For this review, take the finished solid that the model builds, in its own axes (mm). Give positions to 0.01 mm unless a question says otherwise; leave off trailing zeros. Write each loop counter-clockwise with the first axis right and the second up, starting at its lowest first coordinate (ties: lowest second). Pieces come first, ordered by that corner, then holes. Notation, with made-up numbers: (58.25, -22) -> (77.25, -22) arc R4 cw to (77.25, -18) -> close; hole circle Ø9 at (32.25, 35). An arc over 180 degrees is marked (long way). Return JSON: item names as keys, results as strings.
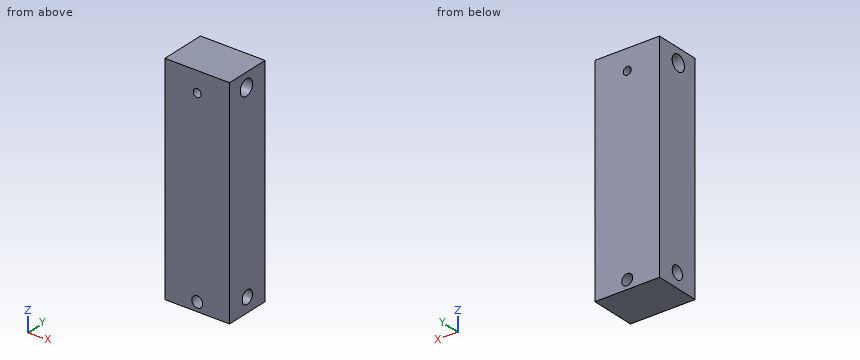
from build123d import *

# Parameters (mm, degrees)
SKETCH_1_W          = 34.660183122
SKETCH_1_H          = 24.57042631
EXTRUDE_1_DEPTH     = 117
SKETCH_2_R          = 2.936506095
SKETCH_2_R_2        = 2.138363717
CUT_EXTRUDE_1_DEPTH = 117
SKETCH_3_R          = 4.242126228
CUT_EXTRUDE_2_DEPTH = 117
SKETCH_4_R          = 3.532728848
CUT_EXTRUDE_3_DEPTH = 50


with BuildPart() as part:
    # 草图1 → 凸台-拉伸1 (new body)
    with BuildSketch(Plane.XY):
        with Locations((17.330091561, 12.285213155)):
            Rectangle(SKETCH_1_W, SKETCH_1_H)
    extrude(amount=EXTRUDE_1_DEPTH)

    # 草图2 → 切除-拉伸1 (cut)
    with BuildSketch(Plane(origin=(0, 24.57042631, 0), x_dir=(1, 0, 0), z_dir=(0, 1, 0))):
        with Locations((17.330091561, -4.778141965)):
            Circle(SKETCH_2_R)
        with Locations((17.330091561, -106.034000041)):
            Circle(SKETCH_2_R_2)
    extrude(amount=-CUT_EXTRUDE_1_DEPTH, mode=Mode.SUBTRACT)

    # 草图3 → 切除-拉伸2 (cut)
    with BuildSketch(Plane.ZY):
        with Locations((109.575398108, 11.633186796)):
            Circle(SKETCH_3_R)
    extrude(amount=-CUT_EXTRUDE_2_DEPTH, mode=Mode.SUBTRACT)

    # 草图4 → 切除-拉伸3 (cut)
    with BuildSketch(Plane(origin=(34.660183122, 0, 0), x_dir=(0, 0, -1), z_dir=(1, 0, 0))):
        with Locations((-7.685412436, 12.285213155)):
            Circle(SKETCH_4_R)
    extrude(amount=-CUT_EXTRUDE_3_DEPTH, mode=Mode.SUBTRACT)


solid = part.part
1. For pin 1 (4 mm diameter, centred on x = 17.33, z = 106.03, fed in from +Y), flat-tipped, find the tip position at first contact; note if it passes through.
Results found:
{"pin 1": "passes through"}
2. To check wall thickness, follow probe 1 along Z at (x, y) = (13.5, 12); probe 2 along Z at (x, y) = (17.5, 23.25); probe 3 along X at (y, z) = (7.25, 5.5). State the ranges of each line that lie inside material, in increasing order.
Results found:
{"probe 1": "z = 0 to 4.16, 11.21 to 105.35, 113.8 to 117", "probe 2": "z = 0 to 1.85, 7.71 to 103.9, 108.17 to 117", "probe 3": "x = 0 to 14.48, 20.18 to 34.66"}
3. Add section A-A, the plane x = 28. State the section outline as (y, z) points, plus the area to 3 significant figures.
Results found:
{"outline": "(0, 0) -> (24.57, 0) -> (24.57, 117) -> (0, 117) -> close; hole circle Ø8.48 at (11.63, 109.58); hole circle Ø7.07 at (12.29, 7.69)", "area": "2,780 mm²"}
